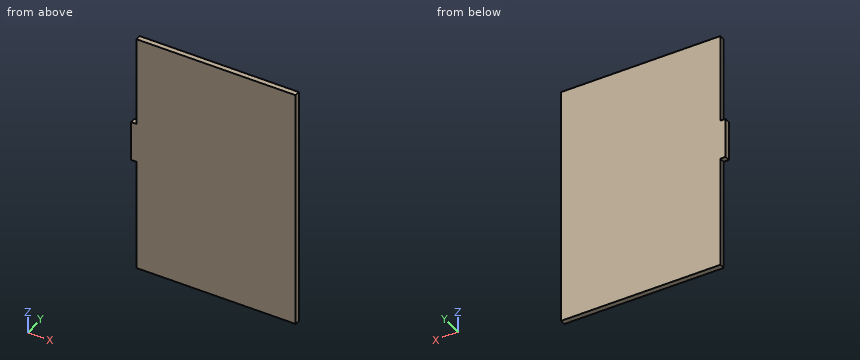
```python
from build123d import *

# Parameters (mm, degrees)
BOSS_EXTRUDE1_DEPTH = 459.74
SKETCH3_W           = 117.668752198
SKETCH3_H           = 459.74
CUT_EXTRUDE1_DEPTH  = 10
SKETCH4_W           = 9.725175386
SKETCH4_H           = 170.179985068
SKETCH4_H_2         = 213.362507046
CUT_EXTRUDE3_DEPTH  = 63


with BuildPart() as part:
    # Sketch1 → Boss-Extrude1 (new body)
    with BuildSketch(Plane.XY):
        Polygon((358.121789204, 754.380000017), (137.961261276, 754.380000017), (137.961261276, 744.380000017), (562.803601281, 744.380000017), (562.803601281, 754.380000017), align=None)
    extrude(amount=BOSS_EXTRUDE1_DEPTH)

    # Sketch3 → Cut-Extrude1 (cut)
    with BuildSketch(Plane.XZ.offset(-744.380000017)):
        with Locations((196.795637375, 229.87)):
            Rectangle(SKETCH3_W, SKETCH3_H)
    extrude(amount=-CUT_EXTRUDE1_DEPTH, mode=Mode.SUBTRACT)

    # Sketch4 → Cut-Extrude3 (cut)
    with BuildSketch(Plane(origin=(0, 754.380000017, 0), x_dir=(1, 0, 0), z_dir=(0, 1, 0))):
        with Locations((260.492601167, -374.650007466)):
            Rectangle(SKETCH4_W, SKETCH4_H)
        with Locations((260.492601167, -106.681253523)):
            Rectangle(SKETCH4_W, SKETCH4_H_2)
    extrude(amount=-CUT_EXTRUDE3_DEPTH, mode=Mode.SUBTRACT)


solid = part.part
```
Verification items for the finished model (mm, model axes). Coordinates: 2 decimals unless noted, no trailing zeros. Write each loop counter-clockwise with the first axis right and the second up, starting at its lowest first coordinate (ties: lowest second). Pieces come first, ordered by that corner, then holes. Notation, with made-up numbers: (6.5, 67) - (53.5, 67) arc R22 cw to (53.5, 104) - close; hole circle Ø9 at (50.25, -12). An arc over 180 degrees is marked (long way). Write item = value, one per line.
Q1. Cross-section at A-A (y = 747.75). Enter the section's corners in (x, z).
Answer:
outline = (255.63, 213.36) - (265.36, 213.36) - (265.36, 0) - (562.8, 0) - (562.8, 459.74) - (265.36, 459.74) - (265.36, 289.56) - (255.63, 289.56) - close
Q2. Go/stop test with flat-tipped pins: pin 1 Ø2 at (y, z) = (747.5, 206) entering from -X; pin 2 Ø3 at (x, y) = (260, 747.5) entering from -Z. Record where each tip stops, or that it passes through.
Answer:
pin_1 = 265.36
pin_2 = 213.36
Q3. Material ranges on L1, parallel to X at y = 750.5, z = 435.5, recorded low to high. Write a range as from..to.
Answer:
L1 = 265.36..562.8
Q4. Cross-section at B-B (z = 394). Enter the section's corners in (x, y).
Answer:
outline = (265.36, 744.38) - (562.8, 744.38) - (562.8, 754.38) - (265.36, 754.38) - close
